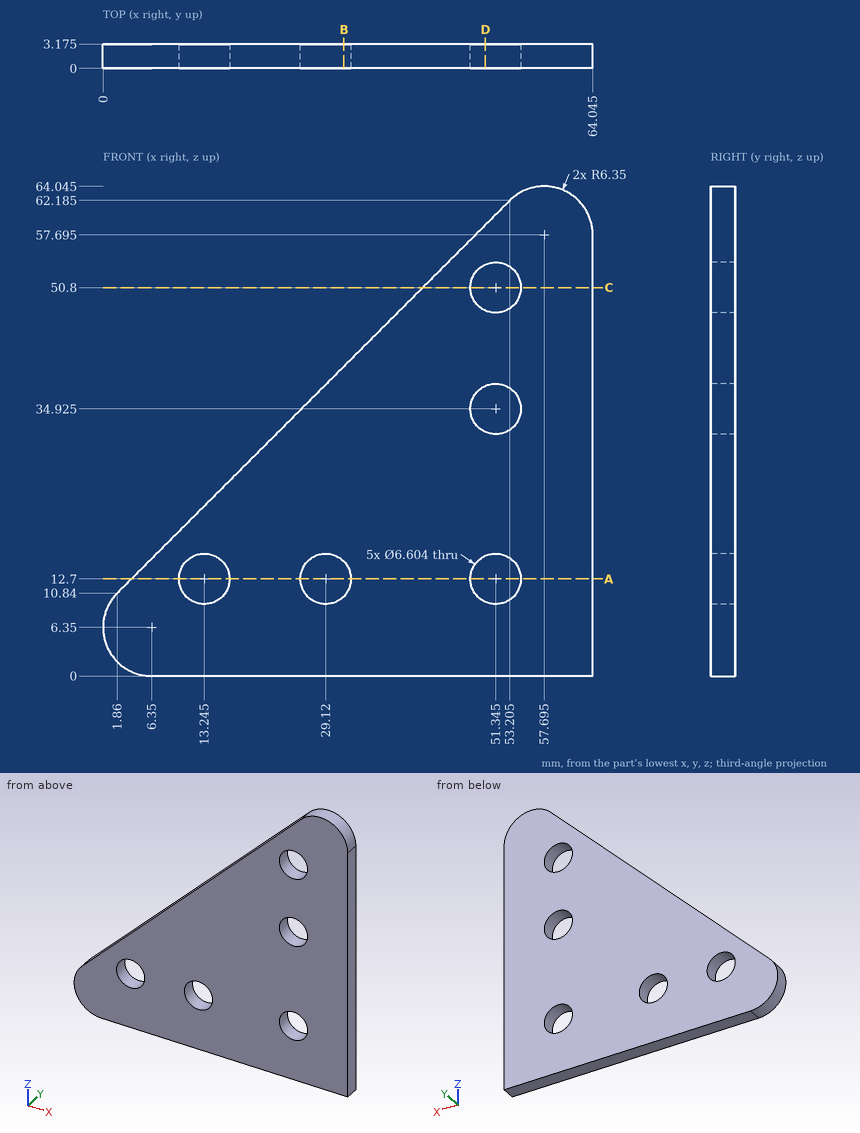
Job drawing, mm, ordinate dimensions from the low corner. One solid piece. Round coordinates to 2 decimals unless told otherwise and drop trailing zeros. Loops run counter-clockwise (first coordinate to the right, second up) from the corner with the lowest first, then second, coordinate; pieces in that order, holes last.
Item 1: Cut at B-B, the plane x = 31.5. Give the cut face in (y, z) (1 decimal), then the cut area to 3 significant figures.
Item 2: Cut at C-C, the plane z = 50.8. Give the cut face in (x, y) (1 decimal), then the cut area to 3 significant figures.
Item 3: Drill centre lines: line 1 (Z direction, x = 51.5, y = 1.1) (1 decimal); line 2 (Z direction, x = 51, y = 2.5) (1 decimal); line 3 (X direction, y = 0.45, z = 33) (1 decimal). Where is each one in solid material? Low to high.
Item 4: Cut at D-D, the plane x = 50. Give the cut face in (y, z) (1 decimal).
Item 5: Cut at A-A, the plane z = 12.7. Give the cut face in (x, y) (1 decimal).
Item 6: Drop flat-ended pins along their axis: P1, Ø6, axis at x = 51.34, z = 34.92, coming from the +Y side (3 decimals); P2, Ø1, axis at x = 13, y = 0.5, coming from the +Z side. Give the stop position or say it passes through.
A:
1. outline: (0, 0) - (3.2, 0) - (3.2, 10.4) - (0, 10.4) - close; (0, 15) - (3.2, 15) - (3.2, 40.5) - (0, 40.5) - close
1. area: 114 mm2
2. outline: (41.8, 0) - (48, 0) - (48, 3.2) - (41.8, 3.2) - close; (54.6, 0) - (64, 0) - (64, 3.2) - (54.6, 3.2) - close
2. area: 49.6 mm2
3. line 1: z = 0 to 9.4, 16 to 31.6, 38.2 to 47.5, 54.1 to 60.5
3. line 2: z = 0 to 9.4, 16 to 31.6, 38.2 to 47.5, 54.1 to 60
3. line 3: x = 24 to 48.7, 54 to 64
4. outline: (0, 0) - (3.2, 0) - (3.2, 9.7) - (0, 9.7) - close; (0, 15.7) - (3.2, 15.7) - (3.2, 31.9) - (0, 31.9) - close; (0, 37.9) - (3.2, 37.9) - (3.2, 47.8) - (0, 47.8) - close; (0, 53.8) - (3.2, 53.8) - (3.2, 59) - (0, 59) - close
5. outline: (3.7, 0) - (9.9, 0) - (9.9, 3.2) - (3.7, 3.2) - close; (16.5, 0) - (25.8, 0) - (25.8, 3.2) - (16.5, 3.2) - close; (32.4, 0) - (48, 0) - (48, 3.2) - (32.4, 3.2) - close; (54.6, 0) - (64, 0) - (64, 3.2) - (54.6, 3.2) - close
6. P1: passes through
6. P2: stops at z = 22.48
